from build123d import *

# Parameters (mm, degrees)
SKETCH1_W                       = 38.1
SKETCH1_H                       = 25.4
BOSS_EXTRUDE1_DEPTH             = 6.35
SKETCH3_W                       = 38.1
SKETCH3_H                       = 13.97
CUT_EXTRUDE1_DEPTH              = 2.1844
SKETCH4_R                       = 1.27
CUT_EXTRUDE2_DEPTH              = 24.271113496
SKETCH6_W                       = 19.05
SKETCH6_H                       = 19.05
CUT_EXTRUDE5_DEPTH              = 24.759524406
SKETCH7_W                       = 31.75
SKETCH7_H                       = 2.0828
CUT_EXTRUDE6_DEPTH              = 12.7
CUT_EXTRUDE9_REACH              = 25.271
SKETCH10_R                      = 1.5
SKETCH15_W                      = 6.263340786
SKETCH15_H                      = 2.0828
CUT_EXTRUDE14_DEPTH             = 1.27
FILLET7_R                       = 1.27
CHAMFER10_SIZE                  = 6.35
F_8_32_TAPPED_HOLE2_D           = 3.4544
F_8_32_TAPPED_HOLE2_DEPTH       = 6.35
F_8_32_TAPPED_HOLE2_CSINK_D     = 5.08
F_8_32_TAPPED_HOLE2_CSINK_ANGLE = 90
F_8_32_TAPPED_HOLE2_TIP         = 1.037806461
F_8_32_TAPPED_HOLE3_D           = 3.4544
F_8_32_TAPPED_HOLE3_DEPTH       = 6.35
F_8_32_TAPPED_HOLE3_CSINK_D     = 5.08
F_8_32_TAPPED_HOLE3_CSINK_ANGLE = 90
F_8_32_TAPPED_HOLE3_TIP         = 1.037806461


with BuildPart() as part:
    # Sketch1 → Boss-Extrude1 (new body)
    with BuildSketch(Plane.XY):
        Rectangle(SKETCH1_W, SKETCH1_H)
    extrude(amount=-BOSS_EXTRUDE1_DEPTH)

    # Sketch3 → Cut-Extrude1 (cut)
    with BuildSketch(Plane.XY):
        with Locations((0, 5.715)):
            Rectangle(SKETCH3_W, SKETCH3_H)
    extrude(amount=-CUT_EXTRUDE1_DEPTH, mode=Mode.SUBTRACT)

    # Sketch4 → Cut-Extrude2 (cut, through all)
    with BuildSketch(Plane.XY.offset(-2.1844)):
        with Locations((-13, 9.652)):
            Circle(SKETCH4_R)
        with Locations(Location((13, 9.652, 0), (0, 0, 180))):
            Circle(SKETCH4_R)
    extrude(amount=-CUT_EXTRUDE2_DEPTH, mode=Mode.SUBTRACT)

    # Sketch6 → Cut-Extrude5 (cut, through all)
    with BuildSketch(Plane.XY):
        with Locations((0, 9.525)):
            Rectangle(SKETCH6_W, SKETCH6_H)
    extrude(amount=-CUT_EXTRUDE5_DEPTH, mode=Mode.SUBTRACT)

    # Sketch7 → Cut-Extrude6 (cut)
    with BuildSketch(Plane(origin=(0, 12.7, 0), x_dir=(1, 0, 0), z_dir=(0, 1, 0))):
        with Locations((0.006850314, 3.2258)):
            Rectangle(SKETCH7_W, SKETCH7_H)
    extrude(amount=-CUT_EXTRUDE6_DEPTH, mode=Mode.SUBTRACT)

    # Sketch10 → Cut-Extrude9 (cut, up to next)
    with BuildSketch(Plane.XY.offset(-2.1844), mode=Mode.PRIVATE) as cut_extrude9_sk1:
        with Locations((-13, 9.652)):
            Circle(SKETCH10_R)
    cut_extrude9_tool1 = extrude(cut_extrude9_sk1.sketch, amount=-CUT_EXTRUDE9_REACH, mode=Mode.PRIVATE) & part.part
    # Sketch10 → Cut-Extrude9 (cut, up to next)
    with BuildSketch(Plane.XY.offset(-2.1844), mode=Mode.PRIVATE) as cut_extrude9_sk2:
        with Locations((13, 9.652)):
            Circle(SKETCH10_R)
    cut_extrude9_tool2 = extrude(cut_extrude9_sk2.sketch, amount=-CUT_EXTRUDE9_REACH, mode=Mode.PRIVATE) & part.part
    add(cut_extrude9_tool1.solids().sort_by_distance((-13, 9.652, -2.1844))[0], mode=Mode.SUBTRACT)
    add(cut_extrude9_tool2.solids().sort_by_distance((13, 9.652, -2.1844))[0], mode=Mode.SUBTRACT)

    # Sketch15 → Cut-Extrude14 (cut)
    with BuildSketch(Plane(origin=(0, 0, 0), x_dir=(1, 0, 0), z_dir=(0, 1, 0))):
        with Locations((-12.736479293, 3.2258)):
            Rectangle(SKETCH15_W, SKETCH15_H)
        with Locations((12.750179921, 3.2258)):
            Rectangle(SKETCH15_W, SKETCH15_H)
    extrude(amount=-CUT_EXTRUDE14_DEPTH, mode=Mode.SUBTRACT)

    # Fillet7
    fillet7_edges = [part.edges().sort_by_distance(p)[0] for p in [
        (15.881850314, -1.27, -3.2258),
        (-15.868149686, -1.27, -3.2258),
        (-9.525, 0, -5.3086),
        (9.525, 0, -5.3086),
        (-9.6048089, -1.27, -3.2258),
        (9.618509528, -1.27, -3.2258),
    ]]
    fillet(fillet7_edges, radius=FILLET7_R - 0.0001)  # a hair under: the kernel refuses the full size

    # Chamfer10
    chamfer10_edges = [part.edges().sort_by_distance(p)[0] for p in [
        (19.05, -12.7, -3.175),
        (-19.05, -12.7, -3.175),
    ]]
    chamfer(chamfer10_edges, length=CHAMFER10_SIZE)

    # #8-32 Tapped Hole2
    with Locations(Plane(origin=(-12.7, -12.7, 0), x_dir=(-0.7071067811865487, 0.7071067811865465, 0), z_dir=(-0.7071067811865465, -0.7071067811865487, 0))):
        with Locations((4.490128061, 3.175)):
            CounterSinkHole(F_8_32_TAPPED_HOLE2_D / 2, F_8_32_TAPPED_HOLE2_CSINK_D / 2, depth=F_8_32_TAPPED_HOLE2_DEPTH, counter_sink_angle=F_8_32_TAPPED_HOLE2_CSINK_ANGLE)
            with Locations((0, 0, -(F_8_32_TAPPED_HOLE2_DEPTH + F_8_32_TAPPED_HOLE2_TIP / 2))):  # 118° drill point
                Cone(0, F_8_32_TAPPED_HOLE2_D / 2, F_8_32_TAPPED_HOLE2_TIP, mode=Mode.SUBTRACT)

    # #8-32 Tapped Hole3
    with Locations(Plane(origin=(12.7, -12.7, 0), x_dir=(0, 0, -1), z_dir=(0.707106781186549, -0.7071067811865461, 0))):
        with Locations((3.175, 4.490128061)):
            CounterSinkHole(F_8_32_TAPPED_HOLE3_D / 2, F_8_32_TAPPED_HOLE3_CSINK_D / 2, depth=F_8_32_TAPPED_HOLE3_DEPTH, counter_sink_angle=F_8_32_TAPPED_HOLE3_CSINK_ANGLE)
            with Locations((0, 0, -(F_8_32_TAPPED_HOLE3_DEPTH + F_8_32_TAPPED_HOLE3_TIP / 2))):  # 118° drill point
                Cone(0, F_8_32_TAPPED_HOLE3_D / 2, F_8_32_TAPPED_HOLE3_TIP, mode=Mode.SUBTRACT)


solid = part.part
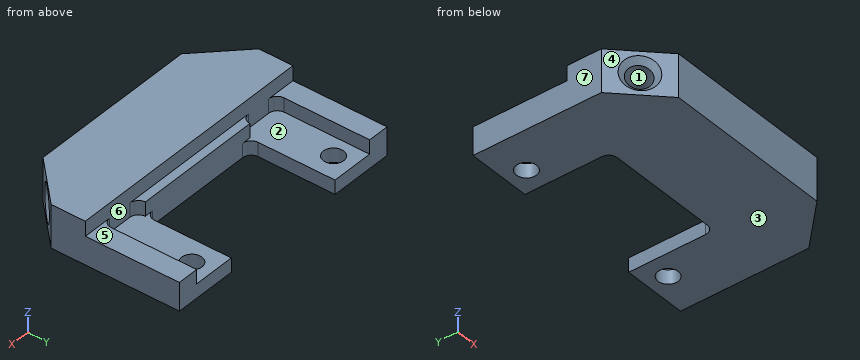
Geometry: final body of the model. Coordinates: model frame, mm. Face numbers are marked on the shaded views. A direction names the side the tool comes from. Round coordinates to 2 decimals unless told otherwise and drop trailing zeros. Order: outer loops, then holes, each group sorted by start corner. A loop starts at its lowest first (then second) coordinate and runs counter-clockwise, first axis right, second up. Notation, with made-up numbers: (45, 24.25) -> (67, 24.25) arc R28 ccw to (67, 53.25) -> close; hole circle Ø2 at (82.5, 39). An arc over 180 degrees is marked (long way). Put each result on its own line as item: value. Start each with the question number.
Q1. Section A-A on y = 4.5. Return the cut outline in (x, z) (3 decimals).
Q2. Line query: probe 1 along X at (y, z) = (8.5, -3); probe 2 along X at (y, z) = (11.75, -5.25) (3 decimals); probe 3 along X at (y, z) = (9, -5.5) (3 decimals). Output: solid intervals per line, ascending.
Q3. Pull-direction query (Z, two-part tool) for the marked faces 1, 2, 3 and 4; classes: +Z half, -Z half, draft (parallel to the pull), parting line (faces both ways), or undercut.
Q4. First-contact query: pin 1 (6 mm diameter, centred on x = 13.5, y = 6.5, fed in from +Z); pin 2 (3 mm diameter, centred on x = 8.5, z = -2.5, fed in from +Y); pin 3 (3.5 mm diameter, centred on x = -13, y = 9.652, fed in from +Z). Flat tips, straight axial feed; report the tip coordinate or a pass-through.
Q5. Reachability of the marked faces 5, 6 and 7 from +Z, -Z, +X, -X, +Y, -Y: full face, straight path, thin tool, end or side. Return the list, or none.
Q6. Section B-B on x = 4. Return the cut outline in (y, z), and give its area (3 significant figures).
Q7. Section C-C on y = -0.5. Return the cut outline in (x, z), and give its area (3 significant figures).
Ans:
1. outline: (-19.05, -6.35) -> (-9.525, -6.35) -> (-9.525, -4.267) -> (-15.868, -4.267) -> (-15.868, -2.184) -> (-19.05, -2.184) -> close; (9.525, -6.35) -> (19.05, -6.35) -> (19.05, -2.184) -> (15.882, -2.184) -> (15.882, -4.267) -> (9.525, -4.267) -> close
2. probe 1: x = -19.05 to -15.87, 15.88 to 19.05
2. probe 2: x = -19.05 to -9.525, 9.525 to 19.05
2. probe 3: x = -19.05 to -14.351, -11.649 to -9.525, 9.525 to 11.649, 14.351 to 19.05
3. face 1: undercut
3. face 2: +Z half
3. face 3: -Z half
3. face 4: draft
4. pin 1: stops at z = -2.18
4. pin 2: stops at y = 0
4. pin 3: stops at z = -4.27
5. face 5: +Z, +X, -X, +Y
5. face 6: +Z, +Y
5. face 7: +Z, -Z, -X, +Y, -Y
6. outline: (-12.7, -6.35) -> (0, -6.35) -> (0, -2.18) -> (-1.27, -2.18) -> (-1.27, 0) -> (-12.7, 0) -> close
6. area: 77.9 mm2
7. outline: (-19.05, -6.35) -> (19.05, -6.35) -> (19.05, -2.18) -> (15.78, -2.18) -> (15.78, -4.27) -> (9.72, -4.27) -> (9.72, -2.18) -> (-9.71, -2.18) -> (-9.71, -4.27) -> (-15.77, -4.27) -> (-15.77, -2.18) -> (-19.05, -2.18) -> close
7. area: 133 mm2
